Model file for the job. Use its own axes, mm. A direction names the side the tool comes from. Round coordinates to 2 decimals unless told otherwise and drop trailing zeros. Order: outer loops, then holes, each group sorted by start corner. A loop starts at its lowest first (then second) coordinate and runs counter-clockwise, first axis right, second up. Notation, with made-up numbers: (-32.5, 7.25) - (24.5, 7.25) arc R29 cw to (24.5, 43.25) - close; hole circle Ø11 at (14.25, 45.25). An arc over 180 degrees is marked (long way). Answer as CSV lines item,"result". Start each with the question number.
1. Band-saw the part on A-A on x = 26.5. List the corners of the cut face in (y, z).
2. Band-saw the part on C-C on y = 43.5. List the corners of the cut face in (x, z).
3. Band-saw the part on B-B on z = 30. List the corners of the cut face in (x, y).
4. 3-axis set-ups, long thin cutter, end or side, ignore diameter. For faces 1 (the face through (3, 16, 9)), 2 (the face through (24.726, 1.972, 30.923)), 3 (the face through (25, 5, 13.101)): which of +Z, -Z, +X, -X, +Y, -Y reach the whole face in a straight line?
5. Band-saw the part on D-D on y = 54.5. List the corners of the cut face in (x, z).
6. Pin check, flat tips, straight feed: pin 1 Ø0.6 at (y, z) = (5, 42) entering from +X; pin 2 Ø10 at (x, z) = (27, 34.5) entering from +Y; pin 3 Ø1 at (x, y) = (1, 5) entering from +Z. Stop position of each tip, or through.
7. Pull direction X, two halves, no side cores. Call faces 4 (the face through (53, 17, 12)), 5 (the face through (20, 0, 30)), 6 (the face through (44, 32, 4)), 7 (the face through (26, 4, 36)): released by +X, released by -X, zero draft, split by the parting line, or undercut.
8. Wall check: line 1 along X through (y, z) = (2, 30); line 2 along Y through (x, z) = (26.5, 1.7); line 3 along Y through (x, z) = (22.5, 9). Give the ranges that are in metal, low to high. Write a range as [from, to].
```python
from build123d import *

# Parameters (mm, degrees)
ESBO_O1_W                  = 53
ESBO_O1_H                  = 60
RESSALTO_EXTRUS_O1_DEPTH   = 4
ESBO_O2_W                  = 53
ESBO_O2_H                  = 4
RESSALTO_EXTRUS_O2_DEPTH   = 60
ESBO_O5_W                  = 3
ESBO_O5_H                  = 36.373853852
RESSALTO_EXTRUS_O3_DEPTH   = 17
CORTE_EXTRUS_O3_DEPTH      = 53
ESBO_O7_W                  = 26.228570329
ESBO_O7_H                  = 46.898944641
ESBO_O7_W_2                = 20
ESBO_O7_H_2                = 41
RESSALTO_EXTRUS_O4_DEPTH   = 6
CORTE_EXTRUS_O4_DEPTH      = 10
CORTE_EXTRUS_O4_DEPTH_BACK = 21
ESBO_O8_R                  = 2
CORTE_EXTRUS_O6_DEPTH      = 45
CORTE_EXTRUS_O6_DEPTH_BACK = 37
ESBO_O9_R                  = 15.9


# Read off the part's stored shape, not the designer's step: Corte-extrus_o3
with BuildPart() as part:
    # Esbo_o1 → Ressalto-extrus_o1 (new body)
    with BuildSketch(Plane.XY):
        with Locations((26.5, 30)):
            Rectangle(ESBO_O1_W, ESBO_O1_H)
    extrude(amount=RESSALTO_EXTRUS_O1_DEPTH)

    # Esbo_o2 → Ressalto-extrus_o2 (add)
    with BuildSketch(Plane.XY):
        with Locations((26.5, 2)):
            Rectangle(ESBO_O2_W, ESBO_O2_H)
    extrude(amount=RESSALTO_EXTRUS_O2_DEPTH)

    # Esbo_o5 → Ressalto-extrus_o3 (add)
    with BuildSketch(Plane.XY):
        with Locations((1.5, 18.186926926)):
            Rectangle(ESBO_O5_W, ESBO_O5_H)
        with Locations((51.5, 18.186926926)):
            Rectangle(ESBO_O5_W, ESBO_O5_H)
    extrude(amount=RESSALTO_EXTRUS_O3_DEPTH)

    # Corte-extrus_o3 outline → Corte-extrus_o3 (cut)
    with BuildSketch(Plane(origin=(0, 0, 0), x_dir=(0, 0, -1), z_dir=(1, 0, 0))):
        with BuildLine():
            ThreePointArc((-17, 5.226597996), (-13.510052949, 22.056538471), (-4, 36.373853852))
            Line((-4, 36.373853852), (-17, 36.373853852))
            Line((-17, 36.373853852), (-17, 5.226597996))
        make_face()
    extrude(amount=CORTE_EXTRUS_O3_DEPTH, mode=Mode.SUBTRACT)

    # Esbo_o7 → Ressalto-extrus_o4 (add)
    with BuildSketch(Plane(origin=(0, 0, 0), x_dir=(1, 0, 0), z_dir=(0, 1, 0))):
        with Locations((25.531831297, -36.55052768)):
            Rectangle(ESBO_O7_W, ESBO_O7_H)
        with Locations((25.674113589, -36.5)):
            Rectangle(ESBO_O7_W_2, ESBO_O7_H_2, mode=Mode.SUBTRACT)
    extrude(amount=RESSALTO_EXTRUS_O4_DEPTH)

    # Esbo_o8 → Corte-extrus_o4 (cut, two sides: drawn at the far end of the back side and taken through both)
    with BuildSketch(Plane(origin=(0, 0, 0), x_dir=(1, 0, 0), z_dir=(0, 1, 0)).offset(-CORTE_EXTRUS_O4_DEPTH_BACK)):
        with Locations(Location((26.5, -30, 0), (0, 0, 270))):
            Circle(ESBO_O8_R)
    extrude(amount=CORTE_EXTRUS_O4_DEPTH + CORTE_EXTRUS_O4_DEPTH_BACK, mode=Mode.SUBTRACT)

    # Esbo_o9 → Corte-extrus_o6 (cut, two sides: drawn at the far end of the back side and taken through both)
    with BuildSketch(Plane.XY.offset(-CORTE_EXTRUS_O6_DEPTH_BACK)):
        with Locations(Location((26.5, 33.9, 0), (0, 0, 180))):
            Circle(ESBO_O9_R)
    extrude(amount=CORTE_EXTRUS_O6_DEPTH + CORTE_EXTRUS_O6_DEPTH_BACK, mode=Mode.SUBTRACT)


solid = part.part
```
Reply:
1,outline,"(0, 0) - (18, 0) - (18, 4) - (4, 4) - (4, 13.1) - (6, 13.1) - (6, 16) - (4, 16) - (4, 28) - (0, 28) - close; (0, 32) - (4, 32) - (4, 57) - (6, 57) - (6, 60) - (0, 60) - close; (49.8, 0) - (60, 0) - (60, 4) - (49.8, 4) - close"
2,outline,"(0, 0) - (13.83, 0) - (13.83, 4) - (0, 4) - close; (39.17, 0) - (53, 0) - (53, 4) - (39.17, 4) - close"
3,outline,"(0, 0) - (24.5, 0) - (24.5, 4) - (15.67, 4) - (15.67, 6) - (12.42, 6) - (12.42, 4) - (0, 4) - close; (28.5, 0) - (53, 0) - (53, 4) - (38.65, 4) - (38.65, 6) - (35.67, 6) - (35.67, 4) - (28.5, 4) - close"
4,face 1,"+Z, +Y"
4,face 2,"+Y, -Y"
4,face 3,"+Y"
5,outline,"(0, 0) - (53, 0) - (53, 4) - (0, 4) - close"
6,pin 1,"stops at x = 38.65"
6,pin 2,"stops at y = 4"
6,pin 3,"stops at z = 17"
7,face 4,"released by +X"
7,face 5,"zero draft"
7,face 6,"undercut"
7,face 7,"undercut"
8,line 1,"x = [0, 24.5], [28.5, 53]"
8,line 2,"y = [0, 18], [49.8, 60]"
8,line 3,"y = [0, 4]"
